```python
from build123d import *

# Parameters (mm, degrees)
F0_W     = 22.225
F0_H     = 22.225
F0_W_2   = 25.4
F0_H_2   = 25.4
F0_W_3   = 3.175
F0_H_3   = 3.175
F1_DEPTH = 3.175


with BuildPart() as f1:
    # F0 (on Top) → F1 (new body)
    with BuildSketch(Plane.XY):
        with Locations((-49.2125, 49.2125)):
            Rectangle(F0_W, F0_H)
        with Locations((-25.4, 49.2125)):
            Rectangle(F0_W_2, F0_H)
        with Locations((25.4, 49.2125)):
            Rectangle(F0_W_2, F0_H)
        with Locations((49.2125, 49.2125)):
            Rectangle(F0_W, F0_H)
        with Locations((49.2125, 25.4)):
            Rectangle(F0_W, F0_H_2)
        with Locations((25.4, 25.4)):
            Rectangle(F0_W_2, F0_H_2)
        with Locations((0, 25.4)):
            Rectangle(F0_W_2, F0_H_2)
        with Locations((-25.4, 25.4)):
            Rectangle(F0_W_2, F0_H_2)
        with Locations((-49.2125, 25.4)):
            Rectangle(F0_W, F0_H_2)
        with Locations((-49.2125, 0)):
            Rectangle(F0_W, F0_H_2)
        with Locations((-25.4, 0)):
            Rectangle(F0_W_2, F0_H_2)
        Rectangle(F0_W_2, F0_H_2)
        with Locations((25.4, 0)):
            Rectangle(F0_W_2, F0_H_2)
        with Locations((49.2125, 0)):
            Rectangle(F0_W, F0_H_2)
        with Locations((49.2125, -25.4)):
            Rectangle(F0_W, F0_H_2)
        with Locations((25.4, -25.4)):
            Rectangle(F0_W_2, F0_H_2)
        with Locations((0, -25.4)):
            Rectangle(F0_W_2, F0_H_2)
        with Locations((-25.4, -25.4)):
            Rectangle(F0_W_2, F0_H_2)
        with Locations((-49.2125, -25.4)):
            Rectangle(F0_W, F0_H_2)
        with Locations((-49.2125, -49.2125)):
            Rectangle(F0_W, F0_H)
        with Locations((-25.4, -49.2125)):
            Rectangle(F0_W_2, F0_H)
        with Locations((25.4, -49.2125)):
            Rectangle(F0_W_2, F0_H)
        with Locations((49.2125, -49.2125)):
            Rectangle(F0_W, F0_H)
        with Locations((0, 49.2125)):
            Rectangle(F0_W_2, F0_H)
        with Locations((0, -49.2125)):
            Rectangle(F0_W_2, F0_H)
        with Locations((-61.9125, -49.2125)):
            Rectangle(F0_W_3, F0_H)
        with Locations((-61.9125, 0)):
            Rectangle(F0_W_3, F0_H_2)
        with Locations((-61.9125, 49.2125)):
            Rectangle(F0_W_3, F0_H)
        with Locations((61.9125, 49.2125)):
            Rectangle(F0_W_3, F0_H)
        with Locations((61.9125, 0)):
            Rectangle(F0_W_3, F0_H_2)
        with Locations((61.9125, -49.2125)):
            Rectangle(F0_W_3, F0_H)
        with Locations((-25.4, -61.9125)):
            Rectangle(F0_W_2, F0_H_3)
        with Locations((25.4, -61.9125)):
            Rectangle(F0_W_2, F0_H_3)
        with Locations((-25.4, 61.9125)):
            Rectangle(F0_W_2, F0_H_3)
        with Locations((25.4, 61.9125)):
            Rectangle(F0_W_2, F0_H_3)
    extrude(amount=F1_DEPTH)


solid = f1.part
```
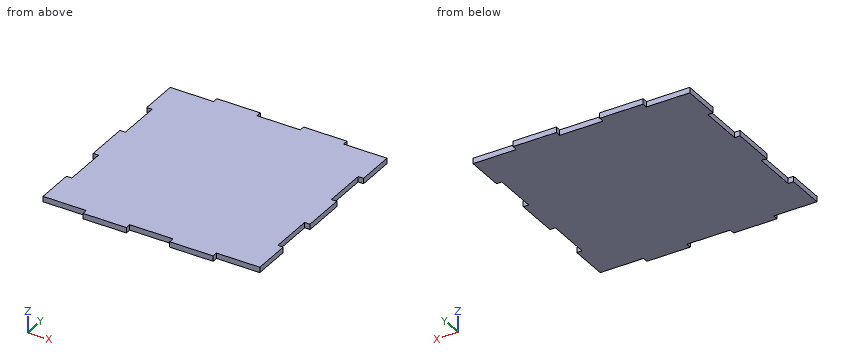
The listing builds one solid part. Answer for the finished solid, in the listing's coordinates (mm). Give positions to 0.01 mm unless a question says otherwise; leave off trailing zeros. Order: outer loops, then holes, each group sorted by start corner. A loop starts at its lowest first (then second) coordinate and runs counter-clockwise, first axis right, second up. Notation, with made-up numbers: (-25.75, -6.75) -> (26.25, -6.75) arc R27 cw to (26.25, 10.25) -> close; hole circle Ø9 at (12, 49). An arc over 180 degrees is marked (long way). Write each question's results on one line, items separated by ' | '.
Q1. A straight line is drawn through the part: probe 1 along X at (y, z) = (-15, 1.15) (3 decimals). Find the intervals that lie inside material, in ascending order. Write a range as from..to.
Checked values:
probe 1: x = -60.325..60.325
Q2. The part is cut by section A-A, the plane x = 43.5. Give the vertices of the cut face in (y, z) (3 decimals), and give its area (3 significant figures).
Checked values:
outline: (-60.325, 0) -> (60.325, 0) -> (60.325, 3.175) -> (-60.325, 3.175) -> close | area: 383 mm^2
Q3. Each of these flat-tipped pins is pushed along its axis until it touches: P1, Ø1.6, axis at y = -28, z = 1.5, coming from the -X side (3 decimals); P2, Ø1, axis at y = 61.5, z = 1.5, coming from the +X side; P3, Ø1, axis at x = -49, z = 1, coming from the +Y side (3 decimals). Where does it stop, or does it pass through?
Checked values:
P1: stops at x = -60.325 | P2: stops at x = 38.1 | P3: stops at y = 60.325
